Input: part model. Units: mm. Frame: model coordinates. Face numbers are marked on the shaded views. A direction names the side the tool comes from. Coordinates: 2 decimals unless noted, no trailing zeros. Loops run counter-clockwise (first coordinate to the right, second up) from the corner with the lowest first, then second, coordinate; pieces in that order, holes last.
Item 1: Section D-D on z = 19. Return loops of the section in (x, y), and give its area (3 significant figures).
Item 2: Ray query, line 1 along Y through (x, z) = (-15, 2.6); line 2 along X through (y, z) = (13.5, 8.25). Return the intervals inside material, ascending.
Item 3: Pull-direction query (Y, two-part tool) for the marked faces 1, 2 and 3; classes: released by +Y, released by -Y, zero draft, split by the parting line, or undercut.
Item 4: Reachability of the marked faces 4 and 5 from +Z, -Z, +X, -X, +Y, -Y: full face, straight path, thin tool, end or side. Return the list, or none.
Item 5: Section C-C on x = -4.25. Return loops of the section in (y, z), and give its area (3 significant figures).
Item 6: Section A-A on x = -15. Return loops of the section in (y, z).
Item 7: Contact query for flat-ended pins moving along their axis: P1, Ø8, axis at x = -17.5, z = 11, coming from the +Y side; P2, Ø2.5, axis at x = -15, y = 15, coming from the -Z side; P3, Ø12.5, axis at y = 14, z = 18.5, coming from the -X side. Output: stop coordinate, or through.
Item 8: Section B-B on z = 15. Return loops of the section in (x, y), and give its area (3 significant figures).
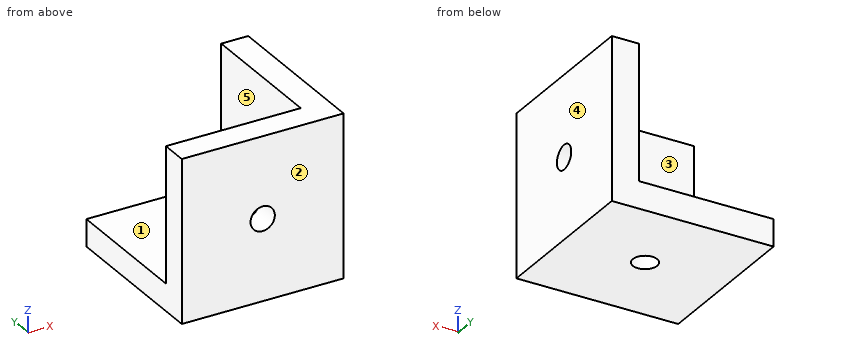
```python
from build123d import *

# Parameters (mm, degrees)
ESBO_O1_W                         = 30
ESBO_O1_H                         = 30
RESSALTO_EXTRUS_O1_DEPTH          = 30
ESBO_O3_W                         = 25
ESBO_O3_H                         = 25
CORTE_EXTRUS_O2_DEPTH             = 25
FURO_COM_FOLGA_DE_M41_D           = 4.5
FURO_COM_FOLGA_DE_M41_ON_FACE_2_D = 4.5
FURO_COM_FOLGA_DE_M41_ON_FACE_3_D = 4.5


with BuildPart() as part:
    # Esboço1 → Ressalto-extrusão1 (new body)
    with BuildSketch(Plane.XY):
        with Locations((-15, 15)):
            Rectangle(ESBO_O1_W, ESBO_O1_H)
    extrude(amount=RESSALTO_EXTRUS_O1_DEPTH)

    # Esboço3 → Corte-extrusão2 (cut)
    with BuildSketch(Plane(origin=(0, 30, 0), x_dir=(1, 0, 0), z_dir=(0, 1, 0))):
        with Locations((-17.5, -17.5)):
            Rectangle(ESBO_O3_W, ESBO_O3_H)
    extrude(amount=-CORTE_EXTRUS_O2_DEPTH, mode=Mode.SUBTRACT)

    # Furo com folga de M41 (through all)
    with Locations(Plane(origin=(-5, 15, 15), x_dir=(0, 0, -1), z_dir=(-1, 0, 0))):
        with Locations((0, 0)):
            Hole(FURO_COM_FOLGA_DE_M41_D / 2)

    # Furo com folga de M41 on face 2 (through all)
    with Locations(Plane(origin=(-15, 15, 5), x_dir=(1, 0, 0), z_dir=(0, 0, 1))):
        with Locations((0, 0)):
            Hole(FURO_COM_FOLGA_DE_M41_ON_FACE_2_D / 2)

    # Furo com folga de M41 on face 3 (through all)
    with Locations(Plane(origin=(-15, 5, 15), x_dir=(0, 0, 1), z_dir=(0, 1, 0))):
        with Locations((0, 0)):
            Hole(FURO_COM_FOLGA_DE_M41_ON_FACE_3_D / 2)


solid = part.part
```
Results found:
1. outline: (-30, 0) - (0, 0) - (0, 30) - (-5, 30) - (-5, 5) - (-30, 5) - close
1. area: 275 mm2
2. line 1: y = 0 to 12.75, 17.25 to 30
2. line 2: x = -5 to 0
3. face 1: zero draft
3. face 2: released by -Y
3. face 3: released by +Y
4. face 4: +Z, -Z, +X, +Y, -Y
4. face 5: +Z, -X, +Y
5. outline: (0, 0) - (30, 0) - (30, 30) - (0, 30) - close; hole circle Ø4.5 at (15, 15)
5. area: 884 mm2
6. outline: (0, 0) - (12.75, 0) - (12.75, 5) - (5, 5) - (5, 12.75) - (0, 12.75) - close; (0, 17.25) - (5, 17.25) - (5, 30) - (0, 30) - close; (17.25, 0) - (30, 0) - (30, 5) - (17.25, 5) - close
7. P1: stops at y = 5
7. P2: passes through
7. P3: stops at x = -5
8. outline: (-30, 0) - (-17.25, 0) - (-17.25, 5) - (-30, 5) - close; (-12.75, 0) - (0, 0) - (0, 12.75) - (-5, 12.75) - (-5, 5) - (-12.75, 5) - close; (-5, 17.25) - (0, 17.25) - (0, 30) - (-5, 30) - close
8. area: 230 mm2
